Job drawing, mm, ordinate dimensions from the low corner. One solid piece. A direction names the side the tool comes from. Give positions to 0.01 mm unless a question says otherwise; leave off trailing zeros. Write each loop counter-clockwise with the first axis right and the second up, starting at its lowest first coordinate (ties: lowest second). Pieces come first, ordered by that corner, then holes. Notation, with made-up numbers: M 58,17.25 L 95,17.25 A33 ccw 95,46.25 Z; hole C 81.25,13 d1. An arc over 180 degrees is marked long. Answer as CSV lines item,"result". Start each with the question number.
Item 1: Band-saw the part on D-D, the plane z = 7.5. List the corners of the cut face in (x, y).
Item 2: Wall check: L1, parallel to Y at x = 14.7, z = 7.5; L2, parallel to Z at x = 5.75, y = 35. Give the ranges that are in metal, low to high. Write a range as from..to.
Item 3: Two-plate mould, pull along Z, no slides. Class the marked faces 3, 4 and 5: +Z half, -Z half, draft (parallel to the pull), parting line (faces both ways), or undercut.
Item 4: Band-saw the part on A-A, the plane x = 7.5. Count the separate pieces of the cut face and the enclosed holes in it, then the cut area to 3 significant figures.
Item 5: Band-saw the part on B-B, the plane z = 12. List the corners of the cut face in (x, y), then the cut area to 3 significant figures.
Item 6: Band-saw the part on C-C, the plane y = 62. List the corners of the cut face in (x, z), then the cut area to 3 significant figures.
Item 7: 3-axis set-ups, long thin cutter, end or side, ignore diameter. For the marked faces 1 and 2: which of +Z, -Z, +X, -X, +Y, -Y reach the whole face in a straight line?
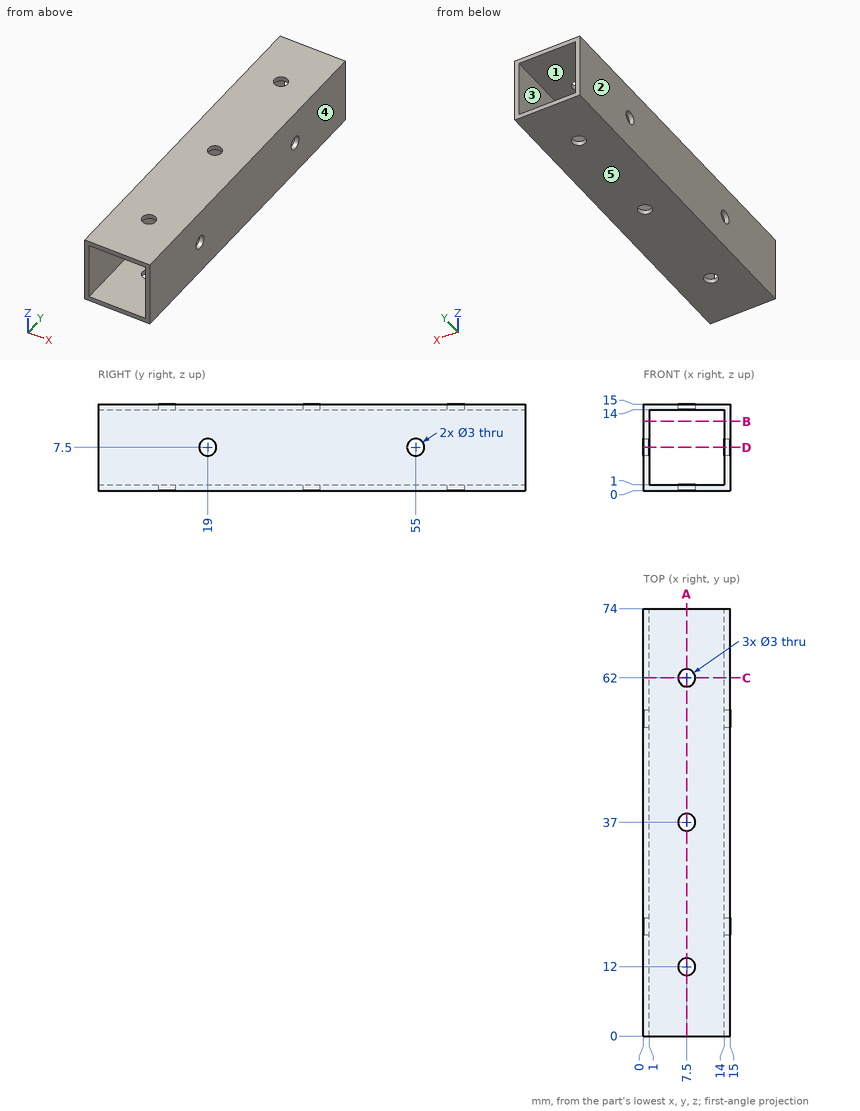
Output:
1,outline,"M 0,0 L 1,0 L 1,17.5 L 0,17.5 Z; M 0,20.5 L 1,20.5 L 1,53.5 L 0,53.5 Z; M 0,56.5 L 1,56.5 L 1,74 L 0,74 Z; M 14,0 L 15,0 L 15,17.5 L 14,17.5 Z; M 14,20.5 L 15,20.5 L 15,53.5 L 14,53.5 Z; M 14,56.5 L 15,56.5 L 15,74 L 14,74 Z"
2,L1,"0..17.5, 20.5..53.5, 56.5..74"
2,L2,"0..1, 14..15"
3,face 3,"undercut"
3,face 4,"draft"
3,face 5,"-Z half"
4,separate pieces,"8"
4,enclosed holes,"0"
4,area,"130 mm²"
5,outline,"M 0,0 L 1,0 L 1,74 L 0,74 Z; M 14,0 L 15,0 L 15,74 L 14,74 Z"
5,area,"148 mm²"
6,outline,"M 0,0 L 6,0 L 6,1 L 1,1 L 1,14 L 6,14 L 6,15 L 0,15 Z; M 9,0 L 15,0 L 15,15 L 9,15 L 9,14 L 14,14 L 14,1 L 9,1 Z"
6,area,"50.0 mm²"
7,face 1,"+Y, -Y"
7,face 2,"+Z, -Z, -X, +Y, -Y"
